Part print with two shaded views. Sizes in mm from the minimum x, y, z corner. A direction names the side the tool comes from. Give positions to 0.01 mm unless a question says otherwise; leave off trailing zeros. Write each loop counter-clockwise with the first axis right and the second up, starting at its lowest first coordinate (ties: lowest second). Pieces come first, ordered by that corner, then holes.
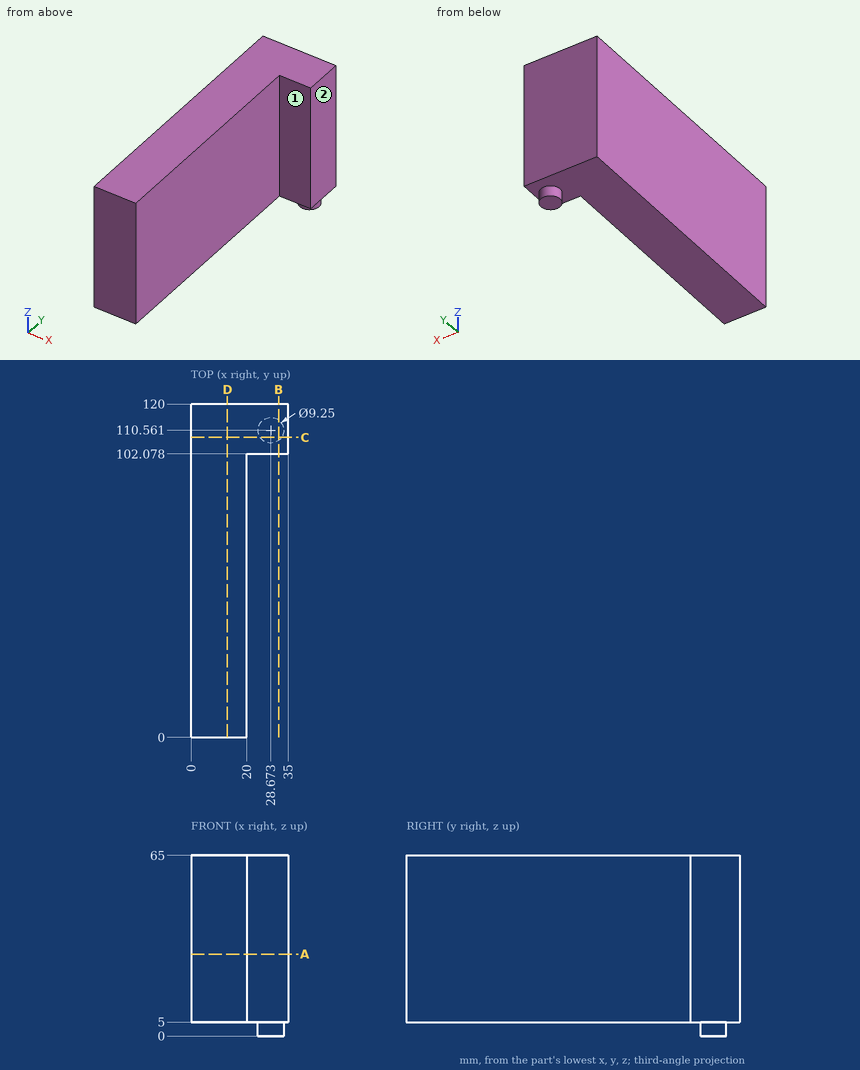
1) Saw through at D-D (x = 13). Write the cut outline in (y, z), and give its area (3 significant figures).
Check result:
outline: (0, 5) - (120, 5) - (120, 65) - (0, 65) - close
area: 7,200 mm2
2) Saw through at C-C (y = 108). Write the cut outline in (x, z).
Check result:
outline: (0, 5) - (24.82, 5) - (24.82, 0) - (32.52, 0) - (32.52, 5) - (35, 5) - (35, 65) - (0, 65) - close
3) Drill centre lines: L1, parallel to X at y = 91.5, z = 47; L2, parallel to Z at x = 6, y = 87; L3, parallel to Y at x = 29, z = 12. Where is each one in solid material? Low to high.
Check result:
L1: x = 0 to 20
L2: z = 5 to 65
L3: y = 102.08 to 120
4) Saw through at B-B (x = 31.5). Write the cut outline in (y, z), and give its area (3 significant figures).
Check result:
outline: (102.08, 5) - (106.9, 5) - (106.9, 0) - (114.22, 0) - (114.22, 5) - (120, 5) - (120, 65) - (102.08, 65) - close
area: 1,110 mm2
5) Saw through at A-A (z = 29.5). Write the cut outline in (x, y).
Check result:
outline: (0, 0) - (20, 0) - (20, 102.08) - (35, 102.08) - (35, 120) - (0, 120) - close
6) Flat gauge pins, fed straight in: P1, Ø12, axis at y = 54.5, z = 7, coming from the +X side; P2, Ø6, axis at y = 82.5, z = 27.5, coming from the -X side; P3, Ø4.5, axis at x = 28, z = 38.5, coming from the -Y side. Where does each tip first touch, or does it go through?
Check result:
P1: stops at x = 20
P2: stops at x = 0
P3: stops at y = 102.08
7) 3-axis set-ups, long thin cutter, end or side, ignore diameter. For the marked faces 1 and 2: which of +Z, -Z, +X, -X, +Y, -Y reach the whole face in a straight line?
Check result:
face 1: +Z, -Z, +X, -Y
face 2: +Z, -Z, +X, +Y, -Y
